Can you work these out from the model? Positions are in its coordinate system, mm. Face numbers are marked on the shaded views. A direction names the side the tool comes from. Give positions to 0.01 mm unless a question says otherwise; leave off trailing zeros. Loops run counter-clockwise (first coordinate to the right, second up) from the corner with the lowest first, then second, coordinate; pieces in that order, holes last. Notation, with made-up numbers: (88, 14.5) -> (139, 14.5) arc R10 cw to (139, 23.5) -> close; hole circle Ø3 at (-8, 52.5). An arc over 180 degrees is marked (long way). Use CSV: the item, a comma, the result in double quotes.
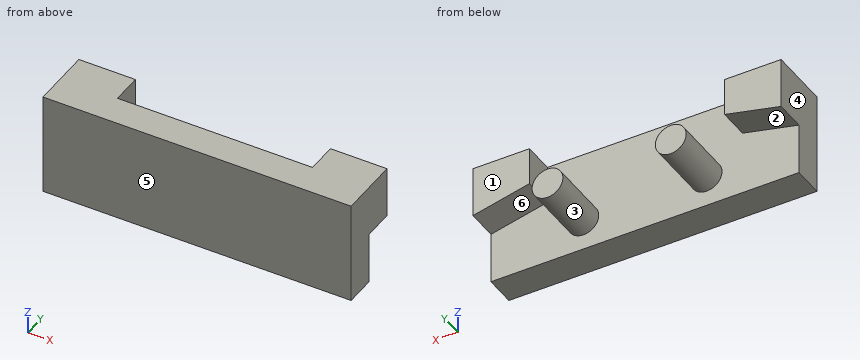
from build123d import *

# Parameters (mm, degrees)
SKETCH2_W             = 30
SKETCH2_H             = 10
BOSS_EXTRUDE2_DEPTH   = 6
CUT_EXTRUDE1_DEPTH    = 3
SKETCH4_4_R           = 1.5
BOSS_EXTRUDE4_DEPTH   = 3
BOSS_EXTRUDE4_2_DEPTH = 3
SKETCH4_5_R           = 1.5
BOSS_EXTRUDE5_DEPTH   = 3


with BuildPart() as part:
    # Sketch2 → Boss-Extrude2 (new body)
    with BuildSketch(Plane(origin=(0, 0, 0), x_dir=(1, 0, 0), z_dir=(0, 1, 0))):
        with Locations((15, -5)):
            Rectangle(SKETCH2_W, SKETCH2_H)
    extrude(amount=BOSS_EXTRUDE2_DEPTH)

    # Sketch4 → Cut-Extrude1 (cut)
    with BuildSketch(Plane(origin=(0, 6, 0), x_dir=(1, 0, 0), z_dir=(0, 1, 0))):
        Polygon((0, -5.027402711), (5.504275855, -6.298164921), (5.504275855, -10), (24.495724145, -10), (24.495724145, -6.298164921), (30, -5.027402711), (30, 0), (0, 0), align=None)
    extrude(amount=-CUT_EXTRUDE1_DEPTH, mode=Mode.SUBTRACT)



with BuildPart() as body_2:
    # Sketch4<4> → Boss-Extrude4 (new body)
    with BuildSketch(Plane(origin=(0, 6, 0), x_dir=(1, 0, 0), z_dir=(0, 1, 0))):
        with Locations((9, -3)):
            Circle(SKETCH4_4_R)
    extrude(amount=BOSS_EXTRUDE4_DEPTH)


with BuildPart() as body_3:
    # Sketch4<4> → Boss-Extrude4 2 (new body)
    with BuildSketch(Plane(origin=(0, 6, 0), x_dir=(1, 0, 0), z_dir=(0, 1, 0))):
        with Locations((21, -3)):
            Circle(SKETCH4_4_R)
    extrude(amount=BOSS_EXTRUDE4_2_DEPTH)


with BuildPart() as part_1:
    add(part.part)

    add(body_2.part)  # Boss-Extrude5 merges body 2

    add(body_3.part)  # Boss-Extrude5 merges body 3
    # Sketch4<5> → Boss-Extrude5 (add)
    with BuildSketch(Plane(origin=(0, 6, 0), x_dir=(1, 0, 0), z_dir=(0, 1, 0))):
        with Locations((9, -3)):
            Circle(SKETCH4_5_R)
        with Locations((21, -3)):
            Circle(SKETCH4_5_R)
    extrude(amount=-BOSS_EXTRUDE5_DEPTH)


solid = part_1.part
(1) We'd pull the mould along X, two halves only. Please class the marked faces 4, 5 and 6: released by +X, released by -X, zero draft, split by the parting line, or undercut.
Answer sheet:
face 4,"released by -X"
face 5,"zero draft"
face 6,"undercut"
(2) Will these pins go through, and if not, where does the flat tip stop? pin 1 Ø5 at (y, z) = (3, 9) entering from -X; pin 2 Ø1 at (x, z) = (17.5, 2.5) entering from +Y; pin 3 Ø4 at (x, y) = (3.5, 7.5) entering from -Z; pin 4 Ø4 at (x, z) = (26.5, 7) entering from +Y.
Answer sheet:
pin 1,"stops at x = 0"
pin 2,"stops at y = 3"
pin 3,"stops at z = 5.53"
pin 4,"stops at y = 6"
(3) If I drill on L1, parallel to Y at x = 23, z = 3; L2, parallel to Y at x = 28.25, z = 6; L3, parallel to X at y = 4.25, z = 4, over which ranges is the centre line in solid material (lowest first)? Write a range as from..to.
Answer sheet:
L1,"y = 0..3"
L2,"y = 0..6"
L3,"x = 7.88..10.12, 19.88..22.12"
(4) If we section it at A-A, the plane y = 4: Write out the boundary of the cut face in (x, z), then the cut area to 3 significant figures.
Answer sheet:
outline,"(0, 5.03) -> (5.5, 6.3) -> (5.5, 10) -> (0, 10) -> close; circle Ø3 at (9, 3); circle Ø3 at (21, 3); (24.5, 6.3) -> (30, 5.03) -> (30, 10) -> (24.5, 10) -> close"
area,"61.9 mm2"
(5) Which directions (+Z, -Z, +X, -X, +Y, -Y) give clear straight access to the entire face, cutting with the end or side of a thin tool? Please do the marked faces 1, 2 and 3.
Answer sheet:
face 1,"+Z, -Z, +X, -X, +Y"
face 2,"-Z, +Y"
face 3,"+Y"
(6) If we section it at C-C, the plane x = 21: Write out the boundary of the cut face in (y, z), then the cut area to 3 significant figures.
Answer sheet:
outline,"(0, 0) -> (3, 0) -> (3, 1.5) -> (9, 1.5) -> (9, 4.5) -> (3, 4.5) -> (3, 10) -> (0, 10) -> close"
area,"48.0 mm2"
(7) If we section it at B-B, the plane z = 3: Write out the boundary of the cut face in (x, y).
Answer sheet:
outline,"(0, 0) -> (30, 0) -> (30, 3) -> (22.5, 3) -> (22.5, 9) -> (19.5, 9) -> (19.5, 3) -> (10.5, 3) -> (10.5, 9) -> (7.5, 9) -> (7.5, 3) -> (0, 3) -> close"
(8) If we section it at D-D, the plane y = 6.75: Write out the boundary of the cut face in (x, z), then the cut area to 3 significant figures.
Answer sheet:
outline,"circle Ø3 at (9, 3); circle Ø3 at (21, 3)"
area,"14.1 mm2"
